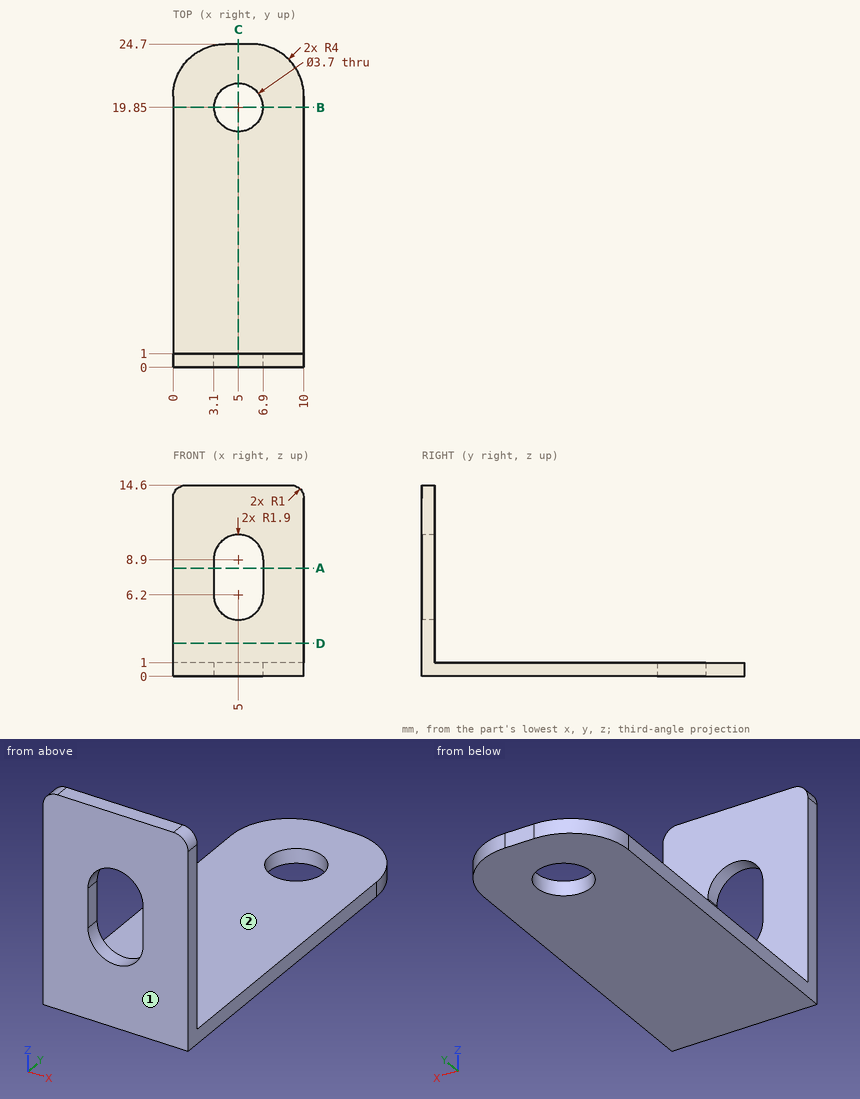
Check sheet for the drawn part. Datum: minimum x, y, z corner. Units: mm. A direction names the side the tool comes from. Round coordinates to 2 decimals unless told otherwise and drop trailing zeros. Loops run counter-clockwise (first coordinate to the right, second up) from the corner with the lowest first, then second, coordinate; pieces in that order, holes last. Notation, with made-up numbers: (72, -4.75) - (129, -4.75) arc R18 cw to (129, 19.25) - close; hole circle Ø1 at (54, 88). An arc over 180 degrees is marked (long way). Write item = value, one per line. Start each with the question number.
1. Depth check by flat-ended pin: pin 1 (5 mm diameter, centred on x = 3, y = 8, fed in from +Z); pin 2 (1 mm diameter, centred on y = 3, z = 9, fed in from +X); pin 3 (5 mm diameter, centred on x = 6.5, z = 9.5, fed in from +Y). Enter the tip coordinate at first touch or a pass-through.
2. Section check D-D on z = 2.5. Enter the section's corners in (x, y), then the cut area to 3 significant figures.
3. Section check C-C on x = 5. Enter the section's corners in (y, z).
4. Set-up check for the marked faces 1 and 2: record each of +Z, -Z, +X, -X, +Y, -Y from which the full face is reachable in a straight line by a thin tool's end or side.
5. Section check B-B on y = 19.85. Enter the section's corners in (x, z), then the cut area to 3 significant figures.
6. Thickness scan on line 1 (Y direction, x = 5, z = 0.7); line 2 (Z direction, x = 5.5, y = 4.25). Record the ranges inside material, lowest first.
7. Section check A-A on z = 8.25. Enter the section's corners in (x, y), then the cut area to 3 significant figures.
Working result:
q1.pin_1 = 1
q1.pin_2 = through
q1.pin_3 = 1
q2.outline = (0, 0) - (10, 0) - (10, 1) - (0, 1) - close
q2.area = 10.0 mm^2
q3.outline = (0, 0) - (18, 0) - (18, 1) - (1, 1) - (1, 4.3) - (0, 4.3) - close; (0, 10.8) - (1, 10.8) - (1, 14.6) - (0, 14.6) - close; (21.7, 0) - (24.7, 0) - (24.7, 1) - (21.7, 1) - close
q4.face_1 = +Z, -Z, +X, -X, -Y
q4.face_2 = +Z, +X, -X, +Y
q5.outline = (0, 0) - (3.15, 0) - (3.15, 1) - (0, 1) - close; (6.85, 0) - (10, 0) - (10, 1) - (6.85, 1) - close
q5.area = 6.30 mm^2
q6.line_1 = 0 to 18, 21.7 to 24.7
q6.line_2 = 0 to 1
q7.outline = (0, 0) - (3.1, 0) - (3.1, 1) - (0, 1) - close; (6.9, 0) - (10, 0) - (10, 1) - (6.9, 1) - close
q7.area = 6.20 mm^2
